from build123d import *

# Parameters (mm, degrees)
F0_R     = 7.175426
F1_DEPTH = 7
F2_R     = 7.175426
F2_R_2   = 1.6
F3_DEPTH = 1.2
F4_R     = 1.5


with BuildPart() as f1:
    # F0 (on Top) → F1 (new body)
    with BuildSketch(Plane.XY):
        Circle(F0_R)
        Polygon((0, -3.175426), (-2.75, -1.587713), (-2.75, 1.587713), (0, 3.175426), (2.75, 1.587713), (2.75, -1.587713), align=None, mode=Mode.SUBTRACT)
    extrude(amount=F1_DEPTH)

    # F2 (on face) → F3 (join)
    with BuildSketch(Plane(origin=(0, 0, 0), x_dir=(1, 0, 0), z_dir=(0, 0, -1))):
        Circle(F2_R)
        Circle(F2_R_2, mode=Mode.SUBTRACT)
    extrude(amount=F3_DEPTH)

    # F4
    f4_edges = [f1.edges().sort_by_distance(p)[0] for p in [
        (-7.175426, 0, 7),
        (-1.375, -2.38157, 7),
        (-2.75, 0, 7),
        (-1.375, 2.38157, 7),
        (1.375, 2.38157, 7),
        (2.75, 0, 7),
        (1.375, -2.38157, 7),
    ]]
    fillet(f4_edges, radius=F4_R)


solid = f1.part
Verification items for the finished model (mm, model axes). A direction names the side the tool comes from. Coordinates: 2 decimals unless noted, no trailing zeros. Order: outer loops, then holes, each group sorted by start corner. A loop starts at its lowest first (then second) coordinate and runs counter-clockwise, first axis right, second up. Notation, with made-up numbers: M 79,22.5 L 91,22.5 A14 ccw 91,43.5 Z; hole C -22,57.25 d3. An arc over 180 degrees is marked long. One line per item, written item: value. Start each with the question number.
Item 1: Sectioned sample at A-A (y = 0). Enter the section's corners in (x, z), then the cut area to 3 significant figures.
Item 2: Sectioned sample at B-B (z = 0.5). Enter the section's corners in (x, y).
Item 3: Mould release check, pull along X, two halves, no side actions. Record for faces 3 (the flat face through (-2.75, 0, 3)), 4 (the cylindrical face through (6.844, -2.155, 2.197)), 5 (the cylindrical face through (-1.27, 0.97, -0.59)), 6 (the flat face through (-2, 0, -1.2)): released by +X, released by -X, zero draft, split by the parting line, or undercut.
Item 4: Scan lines: probe 1 along Y at (x, z) = (0, -0.8); probe 2 along X at (y, z) = (-1, 5.25). Record each from-to range of solid material in increasing order.
Item 5: Access from +Z, -Z, +X, -X, +Y, -Y to the whole of each face (thin tool, end or side, straight path). Record for faces 1 (the cylindrical face through (-3.2, 0.03, 6.57)), 2 (the flat face through (-2, -4, 7)).
Item 6: Gauge pin test, flat ends, axial feed: pin 1 (3 mm diameter, centred on y = 2.5, z = 1.5, fed in from -X); pin 2 (1 mm diameter, centred on y = -5.5, z = 4, fed in from -X); pin 3 (3 mm diameter, centred on y = -3, z = 0.5, fed in from +X). Record the tip position at first contact, or that the pin passes through.
Conclusion:
1. outline: M -7.18,-1.2 L -1.6,-1.2 L -1.6,0 L -2.75,0 L -2.75,5.5 A1.5 ccw -4.25,7 L -5.68,7 A1.5 ccw -7.18,5.5 Z; M 1.6,-1.2 L 7.18,-1.2 L 7.18,5.5 A1.5 ccw 5.68,7 L 4.25,7 A1.5 ccw 2.75,5.5 L 2.75,0 L 1.6,0 Z
1. area: 73.4 mm^2
2. outline: C 0,0 d14.35; hole M -2.75,-1.59 L 0,-3.18 L 2.75,-1.59 L 2.75,1.59 L 0,3.18 L -2.75,1.59 Z
3. face 3: undercut
3. face 4: split by the parting line
3. face 5: undercut
3. face 6: zero draft
4. probe 1: y = -7.18 to -1.6, 1.6 to 7.18
4. probe 2: x = -7.11 to -2.75, 2.75 to 7.11
5. face 1: +Z
5. face 2: +Z, +X, -X, +Y, -Y
6. pin 1: stops at x = -7.11
6. pin 2: stops at x = -5.15
6. pin 3: stops at x = 7.02
